Can you work these out from the model? Positions are in its coordinate system, mm. Coordinates: 2 decimals unless noted, no trailing zeros. Order: outer loops, then holes, each group sorted by start corner. A loop starts at its lowest first (then second) coordinate and runs counter-clockwise, first axis right, second up. Notation, with made-up numbers: (51, -37) -> (91, -37) arc R18 ccw to (91, -32) -> close; hole circle Ø10 at (40, 39.5). An arc over 180 degrees is marked (long way). Answer in a Markdown table with one row per item.
```python
from build123d import *

# Parameters (mm, degrees)
VACIADO1_T  = -5
REDONDEO2_R = 2.5


with BuildPart() as part:
    # Croquis1 → Revolución1 (revolve)
    with BuildSketch(Plane.XY, mode=Mode.PRIVATE) as revoluci_n1_sk:
        Polygon((0, 400), (150, 400), (120, 0), (0, 0), align=None)
    revolve(revoluci_n1_sk.sketch.rotate(Axis((0, 0, 0), (0, 1, 0)), 90), axis=Axis((0, 0, 0), (0, 1, 0)))

    # Vaciado1
    vaciado1_openings = [part.faces().sort_by_distance(p)[0] for p in [
        (0, 400, 0),
    ]]
    offset(amount=VACIADO1_T, openings=vaciado1_openings, kind=Kind.INTERSECTION)

    # Redondeo2
    redondeo2_edges = [part.edges().sort_by_distance(p)[0] for p in [
        (0, 400, 150),
        (0, 400, 144.98595722),
    ]]
    fillet(redondeo2_edges, radius=REDONDEO2_R - 0.0001)  # a hair under: the kernel refuses the full size


solid = part.part
```
(1) We'd pull the mould along Z, two halves only. Please class faces 1 (the conical face through (-128.775, 198.595, 16.908)), 2 (the conical face through (131.488, 195.875, 29.198)), 3 (the flat face through (-2, 0, 2)): +Z half, -Z half, draft (parallel to the pull), parting line (faces both ways), or undercut.
Response values:
| item | result |
|---|---|
| face 1 | undercut |
| face 2 | parting line |
| face 3 | draft |
(2) Suppose I cut it at C-C (y = 215). Please give me the cut outline in (x, z) (3 decimals).
Response values:
| item | result |
|---|---|
| outline | circle Ø272.25 at (0, 0); hole circle Ø262.222 at (0, 0) |
(3) Suppose I cut it at D-D (y = 32). Please give me the cut outline in (x, z), and give its area (3 significant figures).
Response values:
| item | result |
|---|---|
| outline | circle Ø244.8 at (0, 0); hole circle Ø234.77 at (0, 0) |
| area | 3,780 mm2 |
(4) Will these pins go through, and if not, where does the flat tip stop? pin 1 Ø12 at (y, z) = (83, 101.5) entering from +X; pin 2 Ø1.5 at (y, z) = (139.5, 74) entering from -X; pin 3 Ø10 at (y, z) = (226.5, -41.5) entering from +X.
Response values:
| item | result |
|---|---|
| pin 1 | x = 82.57 |
| pin 2 | x = -107.96 |
| pin 3 | x = 132.09 |
(5) I need wall thicknesses on line 1 (Y direction, x = 27, z = 17.5); line 2 (Z direction, x = 124, y = 365); line 3 (Z direction, x = -58, y = 64). Which ranges of each line are inside material? Lowest first, please. Write a range as [from, to].
Response values:
| item | result |
|---|---|
| line 1 | [0, 5] |
| line 2 | [-79.65, -69.93], [69.93, 79.65] |
| line 3 | [-110.5, -104.81], [104.81, 110.5] |
